from build123d import *

# Parameters (mm, degrees)
CUT_EXTRUDE1_DEPTH = 2


with BuildPart() as part:
    # Sketch1 → Revolve1 (revolve)
    with BuildSketch(Plane.XY, mode=Mode.PRIVATE) as revolve1_sk:
        Polygon((0, 0), (3, 0), (3, 4), (2, 4), (2, 13), (1.5, 13), (1.5, 21), (0, 21), align=None)
    revolve(revolve1_sk.sketch.rotate(Axis((0, 21, 0), (0, -1, 0)), 90), axis=Axis((0, 21, 0), (0, -1, 0)))

    # Sketch2 → Cut-Extrude1 (cut)
    with BuildSketch(Plane.XZ):
        Polygon((0, -1.732050808), (1.5, -0.866025404), (1.5, 0.866025404), (0, 1.732050808), (-1.5, 0.866025404), (-1.5, -0.866025404), align=None)
    extrude(amount=-CUT_EXTRUDE1_DEPTH, mode=Mode.SUBTRACT)


solid = part.part
Could you check a few things on this model? Use its own coordinates, in mm. A direction names the side the tool comes from. Give positions to 0.01 mm unless a question says otherwise; leave off trailing zeros. Order: outer loops, then holes, each group sorted by start corner. A loop starts at its lowest first (then second) coordinate and runs counter-clockwise, first axis right, second up. Notation, with made-up numbers: (-24, -21) - (25, -21) arc R24 cw to (25, 7) - close; hole circle Ø7 at (55.25, 47). An arc over 180 degrees is marked (long way). Return JSON: item names as keys, results as strings. Group by question number.
Q1. Please list where these lines run through material, in increasing order: line 1 along X through (y, z) = (1.5, 0); line 2 along X through (y, z) = (16.5, -0.1); line 3 along Y through (x, z) = (-1.1, -2.65). Write a range as [from, to].
Q2. Suppose I cut it at A-A, the plane z = 0. Please give me the cut outline in (x, y).
Q3. Which directions (+Z, -Z, +X, -X, +Y, -Y) give clear straight access to the entire face, cutting with the end or side of a thin tool? Please do faces 1 (the face through (-0.74, 0.986, 1.305)), 2 (the face through (-0.45, 17.06, 1.43)), 3 (the face through (-0.9, 2.03, 2.86)).
Q4. Suppose I cut it at B-B, the plane x = 1.7. Please give me the cut outline in (y, z), and give its area (3 significant figures).
Q5. Will these pins go through, and if not, where does the flat tip stop? pin 1 Ø0.5 at (y, z) = (0.5, 0.5) entering from -X; pin 2 Ø3 at (x, y) = (-0.5, 18.5) entering from -Z; pin 3 Ø3 at (x, y) = (1.5, 6.5) entering from -Z; pin 4 Ø1.9 at (y, z) = (0.5, -0.5) entering from +X.
Q6. Suppose I cut it at D-D, the plane y = 5.5. Please give me the cut outline in (x, z), and give its area (3 significant figures).
Q7. Suppose I cut it at C-C, the plane y = 3. Please give me the cut outline in (x, z).
Q8. Thinking about a two-plate mould opening in X: for faces 4 (the face through (1.3, 0, -1.3)), 5 (the face through (-1.5, 1, 0)), 6 (the face through (2, 9, 0)), 7 (the face through (1.5, 1, 0)), which applies, pulls with the +X half, pulls with the -X half, needs draft (parallel to the pull), parting line crosses it, or undercut?
Resolved:
{
 "1": {"line 1": "x = [-3, -1.5], [1.5, 3]", "line 2": "x = [-1.5, 1.5]", "line 3": "y = [0, 4]"},
 "2": {"outline": "(-3, 0) - (-1.5, 0) - (-1.5, 2) - (1.5, 2) - (1.5, 0) - (3, 0) - (3, 4) - (2, 4) - (2, 13) - (1.5, 13) - (1.5, 21) - (-1.5, 21) - (-1.5, 13) - (-2, 13) - (-2, 4) - (-3, 4) - close"},
 "3": {"face 1": "-Y", "face 2": "+Y", "face 3": "+Y, -Y"},
 "4": {"outline": "(0, -2.47) - (4, -2.47) - (4, -1.05) - (13, -1.05) - (13, 1.05) - (4, 1.05) - (4, 2.47) - (0, 2.47) - close", "area": "38.7 mm2"},
 "5": {"pin 1": "stops at x = -2.99", "pin 2": "stops at z = -1.5", "pin 3": "stops at z = -2", "pin 4": "stops at x = 3"},
 "6": {"outline": "circle Ø4 at (0, 0)", "area": "12.6 mm2"},
 "7": {"outline": "circle Ø6 at (0, 0)"},
 "8": {"face 4": "needs draft", "face 5": "undercut", "face 6": "parting line crosses it", "face 7": "undercut"}
}
